Here's how the part is built. I have some questions about the finished solid (model axes, mm). A direction names the side the tool comes from. Coordinates: 2 decimals unless noted, no trailing zeros. Write each loop counter-clockwise with the first axis right and the second up, starting at its lowest first coordinate (ties: lowest second). Pieces come first, ordered by that corner, then holes.
Item 1: I want a section at A-A (x = -15). Please give me the cut outline in (y, z), and give its area (3 significant figures).
Item 2: For faces 1 (the face through (45.68, 1.97, 16.78)), 2 (the face through (-81.172, 4.507, 12.628)), 3 (the face through (-82, 4, -24)), which set-ups out of +Z, -Z, +X, -X, +Y, -Y let a thin tool reach every point of the face, with its end or its side?
Item 3: I'm going to push a flat-ended pin straight in: P1, Ø2, axis at x = -80.5, z = 14.5, coming from the +Y side. Where does the tip first touch, or does it pass through?
Item 4: If we mould it in two halves opening along Z, with no side actions, what happens to faces 4 (the face through (-14.672, 4.507, 12.628)), 5 (the face through (-18, 0, -12)), 6 (the face through (-14.38, 1.972, 17.787))? For each: pulls with the +Z half, pulls with the -Z half, needs draft (parallel to the pull), parting line crosses it, or undercut.
from build123d import *

# Parameters (mm, degrees)
SKETCH_1_W                   = 140.5
SKETCH_1_H                   = 64
EXTRUDE_1_DEPTH              = 5
HOLE_WIZARD_M3_1_D           = 3.4
HOLE_WIZARD_M3_1_CBORE_D     = 7
HOLE_WIZARD_M3_1_CBORE_DEPTH = 1
SKETCH_4_W                   = 7
SKETCH_4_H                   = 4
CUT_EXTRUDE_1_DEPTH          = 1


with BuildPart() as part:
    # 草图1 → 凸台-拉伸1 (new body)
    with BuildSketch(Plane(origin=(0, 0, 0), x_dir=(1, 0, 0), z_dir=(0, 1, 0))):
        with Locations((-16.998618785, 11.872928177)):
            Rectangle(SKETCH_1_W, SKETCH_1_H)
    extrude(amount=EXTRUDE_1_DEPTH)

    # M3 六角头机械螺钉的柱形沉头孔1 (through all)
    with Locations(Plane(origin=(0, 5, 0), x_dir=(1, 0, 0), z_dir=(0, 1, 0))):
        with Locations((-81.248618785, 25.872928177), (-81.248618785, -16.127071823), (-14.748618785, 25.872928177), (-14.748618785, -16.127071823), (47.251381215, 25.872928177), (47.251381215, -16.127071823)):
            CounterBoreHole(HOLE_WIZARD_M3_1_D / 2, HOLE_WIZARD_M3_1_CBORE_D / 2, HOLE_WIZARD_M3_1_CBORE_DEPTH)

    # 草图4 → 切除-拉伸1 (cut)
    with BuildSketch(Plane(origin=(0, 5, 0), x_dir=(1, 0, 0), z_dir=(0, 1, 0))):
        with Locations((-81.248618785, -18.127071823)):
            Rectangle(SKETCH_4_W, SKETCH_4_H)
        with Locations((-14.748618785, -18.127071823)):
            Rectangle(SKETCH_4_W, SKETCH_4_H)
        with Locations((47.251381215, -18.127071823)):
            Rectangle(SKETCH_4_W, SKETCH_4_H)
    extrude(amount=-CUT_EXTRUDE_1_DEPTH, mode=Mode.SUBTRACT)


solid = part.part
Answer:
1. outline: (0, -43.87) - (5, -43.87) - (5, -29.36) - (4, -29.36) - (4, -27.55) - (0, -27.55) - close; (0, -24.19) - (4, -24.19) - (4, -22.38) - (5, -22.38) - (5, 12.64) - (4, 12.64) - (4, 14.45) - (0, 14.45) - close; (0, 17.81) - (4, 17.81) - (4, 20.13) - (0, 20.13) - close
1. area: 279 mm2
2. face 1: +Y, -Y
2. face 2: +Z, +Y
2. face 3: +Y
3. P1: stops at y = 4
4. face 4: pulls with the +Z half
4. face 5: needs draft
4. face 6: undercut
